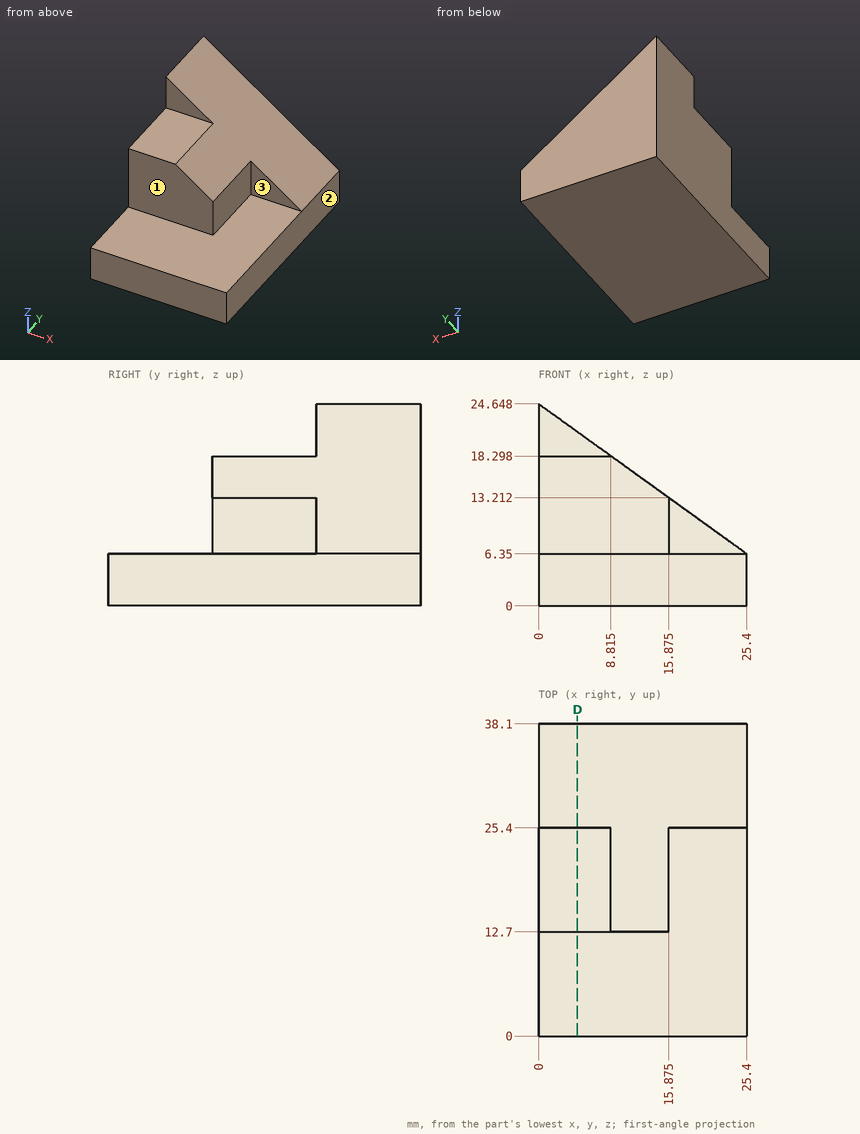
Answer from the drawing. Dimensions are ordinates in mm from the lowest x, y and z of the part. A direction names the side the tool comes from. Give positions to 0.01 mm unless a question says otherwise; leave off trailing zeros. Write each loop counter-clockwise with the first axis right and the second up, starting at its lowest first coordinate (ties: lowest second). Pieces come first, ordered by that corner, then holes. Notation, with made-up numbers: (10, 44) - (16, 44) arc R19 cw to (16, 60) - close; hole circle Ø2 at (5, -26). An arc over 180 degrees is marked (long way). One line per item, written item: value. Start each with the question number.
1. For the marked faces 1, 2 and 3, determine the directions among +Z, -Z, +X, -X, +Y, -Y from which every point of the face is accessible in a straight line to the end or side of a thin tool.
2. Find section D-D (x = 4.75). Write down the section's boundary in (y, z).
3. Consider probe 1 along Z at (x, y) = (7.5, 15.5); probe 2 along Y at (x, z) = (4.5, 11.25); probe 3 along X at (y, z) = (17, 9.75) (1 decimal). Determine where each line is inside the solid, lowest interval first.
4. Given pin 1 (1.5 mm diameter, centred on x = 12.5, y = 5, fed in from +Z); pin 2 (12 mm diameter, centred on x = 5.5, y = 17.5, fed in from +Z); pin 3 (10 mm diameter, centred on x = 6, z = 12, fed in from -Y), each flat-ended and moving along its own axis, determine where each tip first touches the part or whether it passes through.
Geometry results:
1. face 1: +Z, +X, -X, -Y
1. face 2: +Z, -Z, +X, +Y, -Y
1. face 3: +Z, +X, -Y
2. outline: (0, 0) - (38.1, 0) - (38.1, 21.23) - (25.4, 21.23) - (25.4, 18.3) - (12.7, 18.3) - (12.7, 6.35) - (0, 6.35) - close
3. probe 1: 0 to 18.3
3. probe 2: 12.7 to 38.1
3. probe 3: 0 to 15.9
4. pin 1: z = 6.35
4. pin 2: z = 18.3
4. pin 3: y = 12.7
